For this review, take the finished solid that the model builds, in its own axes (mm). Give positions to 0.01 mm unless a question says otherwise; leave off trailing zeros. Loops run counter-clockwise (first coordinate to the right, second up) from the corner with the lowest first, then second, coordinate; pieces in that order, holes last. Notation, with made-up numbers: (63.25, 67.25) - (90.25, 67.25) arc R27 ccw to (90.25, 96.25) - close; hole circle Ø9 at (7, 1). An arc over 180 degrees is marked (long way). Put each result on its own line as item: value. Start each with the question number.
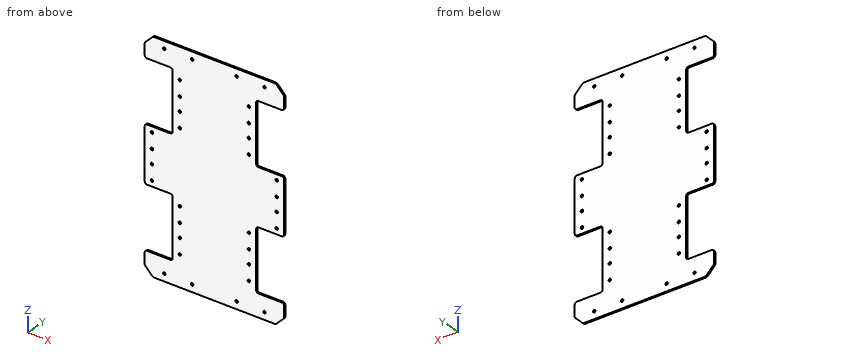
Autodesk Inventor part; units mm, degrees
ref_plane "YZ Plane" through (0, 0, 0) normal (1, 0, 0) x (0, 1, 0)
ref_plane "XZ Plane" through (0, 0, 0) normal (0, 1, 0) x (-1, 0, 0)
ref_plane "XY Plane" through (0, 0, 0) normal (0, 0, 1) x (1, 0, 0)
sketch "Skizze1" plane through (0, 0, 0) normal (0, 1, 0) x (-1, 0, 0)
  line L0 (0, 0) -> (250, 0)
  line L1 (250, 0) -> (250, -400)
  line L2 (250, -400) -> (0, -400)
  line L3 (0, -400) -> (0, 0)
  dimension "d0" = 400
  dimension "d1" = 250
extrude "Extrusion1" add sketch "Skizze1" along normal blind 3
sketch "Skizze7" plane through (0, 3, 0) normal (0, 1, 0) x (1, 0, 0)
  line L0 (-250, 400) -> (-250, 0)
  line L1 (-250, 15) -> (-235, 0)
  line L2 (-250, 0) -> (0, 0)
  line L3 (-250, 15) -> (-250, 0)
  line L4 (-250, 0) -> (-235, 0)
  line L5 (0, 0) -> (0, 400)
  line L6 (0, 0) -> (-15, 0)
  line L7 (-15, 0) -> (0, 15)
  line L8 (-250, 400) -> (-250, 0)
  line L9 (-250, 200) -> (0, 200)
  line L10 (0, 0) -> (0, 400)
  line L11 (-125, 0) -> (-125, 400)
  line L12 (0, 400) -> (-250, 400)
  line L13 (0, 0) -> (0, 15)
  line L14 (-250, 385) -> (-235, 400)
  line L15 (-250, 385) -> (-250, 400)
  line L16 (-250, 400) -> (-235, 400)
  line L17 (0, 400) -> (-15, 400)
  line L18 (-15, 400) -> (0, 385)
  line L19 (0, 400) -> (0, 385)
  point P0 (-200, 30)
  point P1 (0, 30)
  point P2 (-200, 290)
  point P3 (-200, 110)
  point P4 (0, 110)
  point P5 (0, 290)
  point P6 (-235, 400)
  point P7 (-15, 400)
  point P8 (-15, 0)
  dimension "d57" = 15
  dimension "d58" = 15
extrude "Extrusion7" cut sketch "Skizze7" against normal blind 10 contours L12 L14 L0 | L1 L2 L0 | L12 L5 L18 | L5 L2 L7
sketch "Skizze6" plane through (0, 3, 0) normal (0, 1, 0) x (1, 0, 0)
  line L0 (-200, 40) -> (-200, 40)
  line L1 (-250, 0) -> (0, 0)
  line L2 (0, 400) -> (-250, 400)
  line L3 (0, 40) -> (0, 40)
  line L4 (-250, 400) -> (-250, 0)
  line L5 (-250, 250) -> (-200, 250)
  line L6 (-200, 250) -> (-200, 360)
  line L7 (-200, 360) -> (-250, 360)
  line L8 (-250, 360) -> (-250, 250)
  line L9 (-125, 400) -> (-125, 0)
  line L10 (0, 0) -> (0, 400)
  line L11 (0, 200) -> (-250, 200)
  line L12 (0, 400) -> (0, 0)
  line L13 (0, 250) -> (-50, 250)
  line L14 (-50, 250) -> (-50, 360)
  line L15 (-50, 360) -> (0, 360)
  line L16 (-250, 0) -> (-250, 400)
  line L17 (-250, 150) -> (-200, 150)
  line L18 (-200, 150) -> (-200, 40)
  line L19 (-200, 40) -> (-250, 40)
  line L20 (0, 400) -> (0, 0)
  line L21 (-50, 40) -> (0, 40)
  line L22 (-50, 150) -> (-50, 40)
  line L23 (0, 150) -> (-50, 150)
  point P0 (-25, 40)
  point P1 (0, 250)
  point P2 (0, 360)
  point P3 (0, 150)
  dimension "d74" = 110
  dimension "d75" = 40
  dimension "d76" = 50
  dimension "d77" = 110
  dimension "d78" = 50
  dimension "d79" = 110
  dimension "d80" = 50
extrude "Extrusion11" cut sketch "Skizze6" against normal blind 10 contours L4 L17 L18 L19 | L21 L22 L23 L10 | L13 L14 L15 L10 | L4 L7 L6 L5
sketch "Skizze9" plane through (0, 3, 0) normal (0, 1, 0) x (1, 0, 0)
  line L0 (-235, 0) -> (-15, 0)
  line L1 (-125, 0) -> (-125, 400)
  line L2 (-15, 400) -> (-235, 400)
  line L3 (0, 150) -> (0, 250)
  line L4 (0, 200) -> (-250, 200)
  line L5 (-250, 250) -> (-250, 150)
  line L6 (-200, 250) -> (-250, 250)
  line L7 (-237, 250) -> (-237, 150) construction
  circle A0 centre (-237, 240) radius 2.25
  circle A1 centre (-237, 212.5) radius 2.25
  circle A2 centre (-237, 187.5) radius 2.25
  circle A3 centre (-237, 160) radius 2.25
  circle A4 centre (-13, 240) radius 2.25
  circle A5 centre (-13, 212.5) radius 2.25
  circle A6 centre (-13, 187.5) radius 2.25
  circle A7 centre (-13, 160) radius 2.25
  line L8 (-187, 400) -> (-187, 0) construction
  line L9 (-200, 150) -> (-200, 40)
  circle A8 centre (-187, 55) radius 2.25
  circle A9 centre (-187, 82.5) radius 2.25
  circle A10 centre (-187, 107.5) radius 2.25
  circle A11 centre (-187, 135) radius 2.25
  line L10 (-50, 40) -> (-50, 150)
  line L11 (-50, 95) -> (-200, 95) construction
  circle A12 centre (-63, 55) radius 2.25
  circle A13 centre (-63, 82.5) radius 2.25
  circle A14 centre (-63, 107.5) radius 2.25
  circle A15 centre (-63, 135) radius 2.25
  circle A16 centre (-187, 345) radius 2.25
  circle A17 centre (-187, 317.5) radius 2.25
  circle A18 centre (-187, 292.5) radius 2.25
  circle A19 centre (-187, 265) radius 2.25
  circle A20 centre (-63, 345) radius 2.25
  circle A21 centre (-63, 317.5) radius 2.25
  circle A22 centre (-63, 292.5) radius 2.25
  circle A23 centre (-63, 265) radius 2.25
  line L12 (0, 15) -> (0, 40)
  line L13 (0, 13) -> (-250, 13) construction
  line L14 (-250, 40) -> (-250, 15)
  circle A24 centre (-35, 13) radius 2.25
  circle A25 centre (-85, 13) radius 2.25
  circle A26 centre (-165, 13) radius 2.25
  circle A27 centre (-215, 13) radius 2.25
  circle A28 centre (-35, 387) radius 2.25
  circle A29 centre (-85, 387) radius 2.25
  circle A30 centre (-165, 387) radius 2.25
  circle A31 centre (-215, 387) radius 2.25
  point P0 (0, 0)
  dimension "d85" = 13
  dimension "d86" = 4.5
  dimension "d87" = 4.5
  dimension "d88" = 4.5
  dimension "d89" = 4.5
  dimension "d90" = 25
  dimension "d91" = 80
  dimension "d92" = 13
  dimension "d93" = 4.5
  dimension "d94" = 4.5
  dimension "d95" = 4.5
  dimension "d96" = 4.5
  dimension "d97" = 25
  dimension "d98" = 80
  dimension "d99" = 13
  dimension "d100" = 4.5
  dimension "d101" = 4.5
  dimension "d102" = 4.5
  dimension "d103" = 4.5
  dimension "d104" = 80
  dimension "d105" = 180
extrude "Extrusion12" cut sketch "Skizze9" against normal blind 10
fillet "Rundung1" radius 4 24 edges at (-235, 1.5, -400) (-250, 1.5, -385) (-250, 1.5, -360) (-200, 1.5, -360) (-200, 1.5, -250) (-250, 1.5, -250) (-250, 1.5, -150) (-200, 1.5, -150) (-250, 1.5, -40) (-200, 1.5, -40) (-250, 1.5, -15) (-235, 1.5, 0) (-15, 1.5, 0) (0, 1.5, -15) (0, 1.5, -40) (-50, 1.5, -150) (0, 1.5, -150) (-50, 1.5, -40) (0, 1.5, -250) (-50, 1.5, -250) (-15, 1.5, -400) (0, 1.5, -385) (0, 1.5, -360) (-50, 1.5, -360)
equation "\"Biegeradius\" = Stärke"
equation "\"BreiteBiegungsfreistellung\" = Stärke"
equation "\"TiefeBiegungsfreistellung\" = 0.5 * Stärke"
equation "\"GrößeEckenfreistellung\" = 4 * Stärke"
equation "\"MinimalRest\" = 2 * Stärke"
equation "\"Übergangsradius\" = Biegeradius"
equation "\"JacobiRadiusGröße\" = Biegeradius"
equation "\"Abstandsgröße\" = Stärke"
properties part number "Grundgehäuse_01" material "Aluminium 6061"
1) Insertion check: P1, Ø0.9, axis at y = 1.5, z = -306.5, coming from the -X side. The pin has a flat end and moves straight along its axis. Give the tip position at first contact, or say it passes through.
2) Take a section at A-A on y = 1.65. State how many separate pieces and enclosed holes the cut face has, and give its area (3 significant figures).
3) Take a section at B-B on z = -68. State the section outline as (x, y) points, and give its area (3 significant figures).
4) Wall thickness on probe 1 along Z at (x, y) = (-228.5, 1.65); probe 2 along X at (y, z) = (1.9, -212.5); probe 3 along X at (y, z) = (1.2, -292.5): over which ranges is each line inside the solid? List them lowest first.
Answers follow:
1. P1: x = -200
2. separate pieces: 1
2. enclosed holes: 32
2. area: 77,000 mm2
3. outline: (-200, 0) - (-50, 0) - (-50, 3) - (-200, 3) - close
3. area: 450 mm2
4. probe 1: -400 to -360, -250 to -150, -40 to 0
4. probe 2: -250 to -239.25, -234.75 to -15.25, -10.75 to 0
4. probe 3: -200 to -189.25, -184.75 to -65.25, -60.75 to -50
